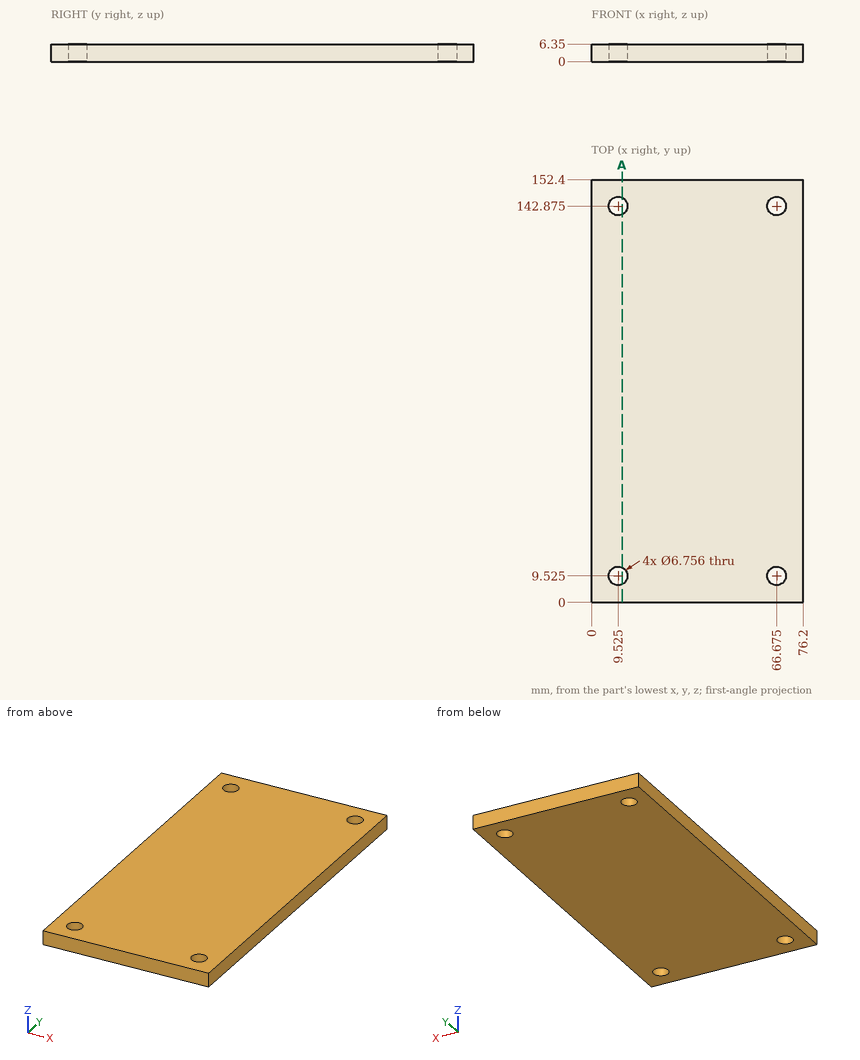
Input: dimensioned drawing with shaded views. Units: mm. Origin: part minimum x, y, z. Give positions to 0.01 mm unless a question says otherwise; leave off trailing zeros. Write each loop counter-clockwise with the first axis right and the second up, starting at its lowest first coordinate (ties: lowest second). Pieces come first, ordered by that corner, then holes.
1. Section query A-A (x = 11). Return the cut outline in (y, z).
2. Material intervals for line 1 along Y through (x, z) = (67.5, 5.5); line 2 along X through (y, z) = (144, 1.75); line 3 along Y through (x, z) = (12, 3) (1 decimal), sorted ascending.
3. First-contact query: pin 1 (5.5 mm diameter, centred on x = 9.525, y = 9.525, fed in from -Z). Flat tip, straight axial feed; report the tip coordinate or a pass-through.
Output values:
1. outline: (0, 0) - (6.49, 0) - (6.49, 6.35) - (0, 6.35) - close; (12.56, 0) - (139.84, 0) - (139.84, 6.35) - (12.56, 6.35) - close; (145.91, 0) - (152.4, 0) - (152.4, 6.35) - (145.91, 6.35) - close
2. line 1: y = 0 to 6.25, 12.8 to 139.6, 146.15 to 152.4
2. line 2: x = 0 to 6.34, 12.71 to 63.49, 69.86 to 76.2
2. line 3: y = 0 to 7.2, 11.8 to 140.6, 145.2 to 152.4
3. pin 1: passes through
